from build123d import *

# Parameters (mm, degrees)
F2_DEPTH = 19.05


with BuildPart() as f2:
    # F1 (on face) → F2 (new body)
    with BuildSketch(Plane.XZ):
        Polygon((-31.75, 44.45), (-31.75, 0), (-31.75, -44.45), (0, -44.45), (31.75, -44.45), (31.75, 0), (31.75, 44.45), (0, 44.45), align=None)
        with BuildLine():
            ThreePointArc((-7.9375, 0), (0, 7.9375), (7.9375, 0))
            ThreePointArc((7.9375, 0), (0, -7.9375), (-7.9375, 0))
        make_face(mode=Mode.SUBTRACT)
    extrude(amount=F2_DEPTH)


solid = f2.part
The listing builds one solid part. Answer for the finished solid, in the listing's coordinates (mm). Give positions to 0.01 mm unless a question says otherwise; leave off trailing zeros. Loops run counter-clockwise (first coordinate to the right, second up) from the corner with the lowest first, then second, coordinate; pieces in that order, holes last. Notation, with made-up numbers: (78.25, 4.25) - (135.25, 4.25) arc R8 ccw to (135.25, 18.25) - close; hole circle Ø1 at (-37, 1.5). An arc over 180 degrees is marked (long way). Write each question's results on one line, items separated by ' | '.
1. Find section A-A, the plane z = 0. Write down the section's boundary in (x, y).
Resolved:
outline: (-31.75, -19.05) - (-7.94, -19.05) - (-7.94, 0) - (-31.75, 0) - close; (7.94, -19.05) - (31.75, -19.05) - (31.75, 0) - (7.94, 0) - close
2. A flat-ended cylindrical pin translates along its axis: P1, Ø14.5, axis at x = 0, z = 0, coming from the +Y side. Find the tip coordinate at first contact, or state that the pin passes through.
Resolved:
P1: passes through
3. Consider probe 1 along Z at (x, y) = (0, -11.75); probe 2 along X at (y, z) = (-11.5, -2.5); probe 3 along X at (y, z) = (-7.25, -4). Determine where each line is inside the solid, lowest interval first. Write a range as from..to.
Resolved:
probe 1: z = -44.45..-7.94, 7.94..44.45 | probe 2: x = -31.75..-7.53, 7.53..31.75 | probe 3: x = -31.75..-6.86, 6.86..31.75
4. For a pull along Y with two mould halves and no side action, classify faces 1 (the face through (0, -19.05, 11)), 2 (the face through (0, 0, 11)), 3 (the face through (0, -9, -44.45)) as +Y half, -Y half, draft (parallel to the pull), parting line (faces both ways), or undercut.
Resolved:
face 1: -Y half | face 2: +Y half | face 3: draft
5. Find section B-B, the plane x = 0. Write down the section's boundary in (y, z), then the cut area to 3 significant figures.
Resolved:
outline: (-19.05, -44.45) - (0, -44.45) - (0, -7.94) - (-19.05, -7.94) - close; (-19.05, 7.94) - (0, 7.94) - (0, 44.45) - (-19.05, 44.45) - close | area: 1,390 mm^2
